```python
from build123d import *

# Parameters (mm, degrees)
ESBO_O1_W                = 320
ESBO_O1_H                = 240
RESSALTO_EXTRUS_O1_DEPTH = 440
CORTE_EXTRUS_O1_DEPTH    = 220
SKETCH4_W                = 320
SKETCH4_H                = 240
BOSS_EXTRUDE2_DEPTH      = 1.2
CUT_EXTRUDE1_DEPTH       = 10
CUT_EXTRUDE2_DEPTH       = 200
SKETCH7_W                = 317.6
SKETCH7_H                = 240
CUT_EXTRUDE3_DEPTH       = 8.8
SKETCH9_W                = 338.812461563
SKETCH9_H                = 258.873896412
CUT_EXTRUDE4_DEPTH       = 1.2


# Read off the part's stored shape, not the designer's step: Corte-extrusão1
with BuildPart() as part:
    # Esboço1 → Ressalto-extrusão1 (new body)
    with BuildSketch(Plane(origin=(0, 0, 0), x_dir=(1, 0, 0), z_dir=(0, 1, 0))):
        Rectangle(ESBO_O1_W, ESBO_O1_H)
    extrude(amount=RESSALTO_EXTRUS_O1_DEPTH)

    # Corte-extrusão1 outline → Corte-extrusão1 (cut)
    with BuildSketch(Plane(origin=(0, 0, 0), x_dir=(1, 0, 0), z_dir=(0, 1, 0))):
        Polygon((158.8, -120), (158.8, -90), (160, -90), (160, 90), (158.8, 90), (158.8, 120), (-158.8, 120), (-158.8, 90), (-160, 90), (-160, -90), (-158.8, -90), (-158.8, -120), align=None)
    extrude(amount=CORTE_EXTRUS_O1_DEPTH, mode=Mode.SUBTRACT)

    # Sketch4 → Boss-Extrude2 (add)
    with BuildSketch(Plane(origin=(0, 440, 0), x_dir=(1, 0, 0), z_dir=(0, 1, 0))):
        Rectangle(SKETCH4_W, SKETCH4_H)
    extrude(amount=BOSS_EXTRUDE2_DEPTH)

    # Esboço5 → Cut-Extrude1 (cut)
    with BuildSketch(Plane.XZ.offset(-220)):
        Polygon((158.8, -90), (158.8, -120), (-158.8, -120), (-158.8, 120), (158.8, 120), align=None)
    extrude(amount=-CUT_EXTRUDE1_DEPTH, mode=Mode.SUBTRACT)

    # Sketch6 → Cut-Extrude2 (cut)
    with BuildSketch(Plane(origin=(0, 231.2, 0), x_dir=(-1, 0, 0), z_dir=(0, -1, 0))):
        Polygon((158.8, -120), (158.8, -90), (160, -90), (160, 90), (158.8, 90), (158.8, 120), (-158.8, 120), (-158.8, 90), (-160, 90), (-160, -90), (-158.8, -90), (-158.8, -120), align=None)
    extrude(amount=-CUT_EXTRUDE2_DEPTH, mode=Mode.SUBTRACT)

    # Sketch7 → Cut-Extrude3 (cut)
    with BuildSketch(Plane(origin=(0, 431.2, 0), x_dir=(-1, 0, 0), z_dir=(0, -1, 0))):
        Rectangle(SKETCH7_W, SKETCH7_H)
    extrude(amount=-CUT_EXTRUDE3_DEPTH, mode=Mode.SUBTRACT)

    # Sketch9 → Cut-Extrude4 (cut)
    with BuildSketch(Plane(origin=(0, 0, 0), x_dir=(-1, 0, 0), z_dir=(0, -1, 0))):
        with Locations((2.117577884, -1.826723931)):
            Rectangle(SKETCH9_W, SKETCH9_H)
    extrude(amount=-CUT_EXTRUDE4_DEPTH, mode=Mode.SUBTRACT)


solid = part.part
```
CAD build for the part. Positions are in the model's coordinates, mm. A direction names the side the tool comes from. Coordinates: 2 decimals unless noted, no trailing zeros. Loops run counter-clockwise (first coordinate to the right, second up) from the corner with the lowest first, then second, coordinate; pieces in that order, holes last. Notation, with made-up numbers: (-27, -13.75) - (-11, -13.75) arc R22 cw to (-11, 17.25) - close; hole circle Ø7 at (80, -35). An arc over 180 degrees is marked (long way). Use CSV: the item, a comma, the result in double quotes. Start each with the question number.
Q1. Cut at C-C, the plane x = -77. List the corners of the cut face in (y, z), then the cut area to 3 significant figures.
Q2. Cut at B-B, the plane z = 80. List the corners of the cut face in (x, y).
Q3. Drop flat-ended pins along their axis: P1, Ø1.3, axis at x = 159.5, z = -40, coming from the -Y side; P2, Ø10, axis at x = 117, z = 36.5, coming from the -Y side. Give the stop position or say it passes through.
Q4. 3-axis set-ups, long thin cutter, end or side, ignore diameter. For faces 1 (the flat face through (160, 220.2, 0.6)), 2 (the flat face through (158.8, 436, -8)), 3 (the flat face through (-158.8, 132, -98)): which of +Z, -Z, +X, -X, +Y, -Y reach the whole face in a straight line?
Q5. Probe probe 1 along Y at (x, z) = (-115, -64); probe 2 along X at (y, z) = (239, -98.5). List the from-to ranges inside material, lowest first. Write a range as from..to.
Q6. Two-plate mould, pull along X, no slides. Class faces 4 (the flat face through (-2, 441.2, -2)), 5 (the flat face through (-160, 220.2, 0.6)), 6 (the flat face through (-158.8, 436, -8)): +X half, -X half, draft (parallel to the pull), parting line (faces both ways), or undercut.
Q7. Cut at A-A, the plane y = 295.5. List the corners of the cut face in (x, z).
Here are the results:
1,outline,"(230, -120) - (231.2, -120) - (231.2, 120) - (230, 120) - close; (440, -120) - (441.2, -120) - (441.2, 120) - (440, 120) - close"
1,area,"576 mm2"
2,outline,"(-160, 220) - (-158.8, 220) - (-158.8, 230) - (158.8, 230) - (158.8, 220) - (160, 220) - (160, 231.2) - (-160, 231.2) - close; (-160, 431.2) - (-158.8, 431.2) - (-158.8, 440) - (158.8, 440) - (158.8, 431.2) - (160, 431.2) - (160, 441.2) - (-160, 441.2) - close"
3,P1,"y = 220"
3,P2,"y = 230"
4,face 1,"+Z, -Z, +X, +Y, -Y"
4,face 2,"+Z, -Z"
4,face 3,"+Z, -Z, -Y"
5,probe 1,"230..231.2, 440..441.2"
5,probe 2,"-160..-158.8, 158.8..160"
6,face 4,"draft"
6,face 5,"-X half"
6,face 6,"undercut"
7,outline,"(-160, -120) - (-158.8, -120) - (-158.8, -90) - (-160, -90) - close; (-160, 90) - (-158.8, 90) - (-158.8, 120) - (-160, 120) - close; (158.8, -120) - (160, -120) - (160, -90) - (158.8, -90) - close; (158.8, 90) - (160, 90) - (160, 120) - (158.8, 120) - close"
